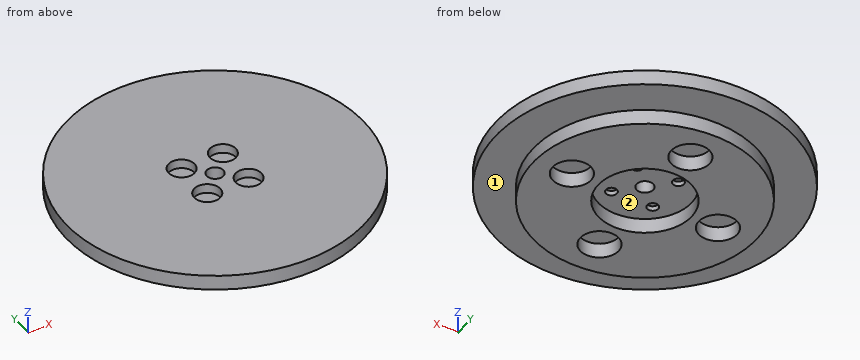
```python
from build123d import *

# Parameters (mm, degrees)
SKETCH1_R           = 30
SKETCH1_R_2         = 12.5
BOSS_EXTRUDE1_DEPTH = 4
SKETCH2_R           = 40
SKETCH2_R_2         = 2.25
SKETCH2_R_3         = 1.5
BOSS_EXTRUDE2_DEPTH = 4
SKETCH3_R           = 3.5
CUT_EXTRUDE1_DEPTH  = 2.5
SKETCH4_R           = 5.15
CUT_EXTRUDE2_DEPTH  = 4
SKETCH5_R           = 3.5
BOSS_EXTRUDE3_DEPTH = 0.2


with BuildPart() as part:
    # Sketch1 → Boss-Extrude1 (new body)
    with BuildSketch(Plane.XY):
        Circle(SKETCH1_R)
        Circle(SKETCH1_R_2, mode=Mode.SUBTRACT)
    extrude(amount=BOSS_EXTRUDE1_DEPTH)

    # Sketch2 → Boss-Extrude2 (add)
    with BuildSketch(Plane.XY.offset(4)):
        Circle(SKETCH2_R)
        Circle(SKETCH2_R_2, mode=Mode.SUBTRACT)
        with Locations((-5.655999742, 5.657708628)):
            Circle(SKETCH2_R_3, mode=Mode.SUBTRACT)
        with Locations((-5.655999742, -5.657708628)):
            Circle(SKETCH2_R_3, mode=Mode.SUBTRACT)
        with Locations((5.655999742, -5.657708628)):
            Circle(SKETCH2_R_3, mode=Mode.SUBTRACT)
        with Locations((5.655999742, 5.657708628)):
            Circle(SKETCH2_R_3, mode=Mode.SUBTRACT)
    extrude(amount=BOSS_EXTRUDE2_DEPTH)

    # Sketch3 → Cut-Extrude1 (cut)
    with BuildSketch(Plane.XY.offset(8)):
        with Locations((-5.655999742, 5.657708628)):
            Circle(SKETCH3_R)
        with Locations((5.655999742, 5.657708628)):
            Circle(SKETCH3_R)
        with Locations((5.655999742, -5.657708628)):
            Circle(SKETCH3_R)
        with Locations((-5.655999742, -5.657708628)):
            Circle(SKETCH3_R)
    extrude(amount=-CUT_EXTRUDE1_DEPTH, mode=Mode.SUBTRACT)

    # Sketch4 → Cut-Extrude2 (cut)
    with BuildSketch(Plane(origin=(0, 0, 0), x_dir=(-1, 0, 0), z_dir=(0, 0, -1))):
        with Locations((-20, 0)):
            Circle(SKETCH4_R)
        with Locations((0, -20)):
            Circle(SKETCH4_R)
        with Locations((20, 0)):
            Circle(SKETCH4_R)
        with Locations((0, 20)):
            Circle(SKETCH4_R)
    extrude(amount=-CUT_EXTRUDE2_DEPTH, mode=Mode.SUBTRACT)

    # Sketch5 → Boss-Extrude3 (add)
    with BuildSketch(Plane.XY.offset(5.5)):
        with Locations((-5.655999742, 5.657708628)):
            Circle(SKETCH5_R)
        with Locations((5.655999742, 5.657708628)):
            Circle(SKETCH5_R)
        with Locations((-5.655999742, -5.657708628)):
            Circle(SKETCH5_R)
        with Locations((5.655999742, -5.657708628)):
            Circle(SKETCH5_R)
    extrude(amount=-BOSS_EXTRUDE3_DEPTH)


solid = part.part
```
Model file for the job. Use its own axes, mm. Face numbers are marked on the shaded views. Round coordinates to 2 decimals unless told otherwise and drop trailing zeros. Write each loop counter-clockwise with the first axis right and the second up, starting at its lowest first coordinate (ties: lowest second). Pieces come first, ordered by that corner, then holes. Notation, with made-up numbers: M -30,-3.5 L -3,-3.5 A21 ccw -3,22.5 Z; hole C 24.5,73 d11. An arc over 180 degrees is marked long. Put each result on its own line as item: value.
Item 1: Cut at C-C (y = 18). List the corners of the cut face in (x, z).
Responses:
outline: M -35.72,4 L -24,4 L -24,0 L -4.75,0 L -4.75,4 L 4.75,4 L 4.75,0 L 24,0 L 24,4 L 35.72,4 L 35.72,8 L -35.72,8 Z
Item 2: Probe L1, parallel to Y at x = 0, z = 1.4; L2, parallel to X at y = -4.5, z = 1.25; L3, parallel to Y at x = -3, z = 7.75. List the from-to ranges inside material, lowest first. Write a range as from..to.
Responses:
L1: -30..-25.15, -14.85..-12.5, 12.5..14.85, 25.15..30
L2: -29.66..-22.5, -17.5..-11.66, 11.66..17.5, 22.5..29.66
L3: -39.89..-7.94, -3.38..3.38, 7.94..39.89
Item 3: Mould opens along X. For the marked faces 1 and 2 say: +X half, -X half, draft (parallel to the pull), parting line (faces both ways), or undercut.
Responses:
face 1: draft
face 2: undercut
Item 4: Cut at A-A (x = 0). List the corners of the cut face in (y, z), and give its area (3 significant figures).
Responses:
outline: M -40,4 L -30,4 L -30,0 L -25.15,0 L -25.15,4 L -14.85,4 L -14.85,0 L -12.5,0 L -12.5,4 L -2.25,4 L -2.25,8 L -40,8 Z; M 2.25,4 L 12.5,4 L 12.5,0 L 14.85,0 L 14.85,4 L 25.15,4 L 25.15,0 L 30,0 L 30,4 L 40,4 L 40,8 L 2.25,8 Z
area: 360 mm²
Item 5: Flat gauge pins, fed straight in: P1, Ø5, axis at x = 18.5, y = 0, coming from the -Z side; P2, Ø1.5, axis at y = 31, z = 1.5, coming from the -X side; P3, Ø3.5, axis at x = -5.66, y = -5.66, coming from the +Z side; P4, Ø0.9, axis at x = 6, y = 6, coming from the -Z side. Where does each tip first touch, or does it go through?
Responses:
P1: z = 4
P2: through
P3: z = 5.5
P4: z = 5.3
Item 6: Cut at B-B (z = 2.75). List the corners of the cut face in (x, y), and give its area (3 significant figures).
Responses:
outline: C 0,0 d60; hole C -20,0 d10.3; hole C 0,0 d25; hole C 0,-20 d10.3; hole C 0,20 d10.3; hole C 20,0 d10.3
area: 2,000 mm²
Item 7: Cut at D-D (x = -22.5). List the corners of the cut face in (y, z).
Responses:
outline: M -33.07,4 L -19.84,4 L -19.84,0 L -4.5,0 L -4.5,4 L 4.5,4 L 4.5,0 L 19.84,0 L 19.84,4 L 33.07,4 L 33.07,8 L -33.07,8 Z
